The listing builds one solid part. Answer for the finished solid, in the listing's coordinates (mm). Face numbers are marked on the shaded views. Coordinates: 2 decimals unless noted, no trailing zeros. Order: outer loops, then holes, each group sorted by start corner. A loop starts at its lowest first (then second) coordinate and runs counter-clockwise, first axis right, second up. Notation, with made-up numbers: (60.25, -12.75) -> (112.25, -12.75) arc R22 cw to (112.25, 10.25) -> close; hole circle Ø9 at (89, 42). An arc over 180 degrees is marked (long way). Return JSON: item names as keys, results as strings.
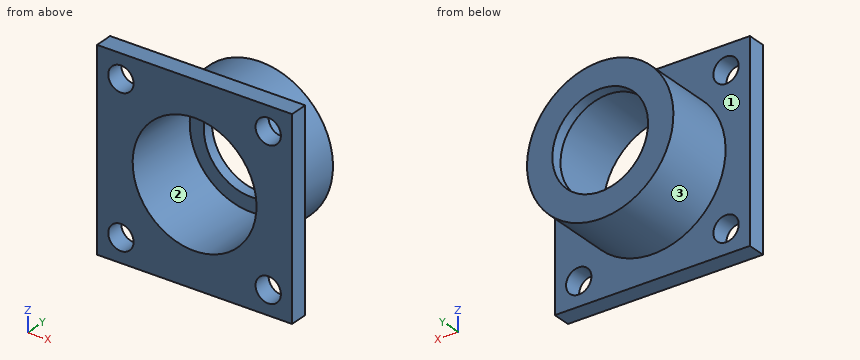
```python
from build123d import *

# Parameters (mm, degrees)
M4_CLEARANCE_HOLE1_D = 4.5
SKETCH5_W            = 85.847558644
SKETCH5_H            = 65.066287946
SKETCH5_W_2          = 34.648232278
SKETCH5_H_2          = 34.648232278
CUT_EXTRUDE2_DEPTH   = 10


with BuildPart() as part:
    # Sketch1 → Revolve1 (revolve)
    with BuildSketch(Plane.XY, mode=Mode.PRIVATE) as revolve1_sk:
        Polygon((-24.5, 0), (-11, 0), (-11, 14), (-8.5, 14), (-8.5, 16), (-13, 16), (-13, 3.2), (-24.5, 3.2), align=None)
    revolve(revolve1_sk.sketch.rotate(Axis((0, 31.465116279, 0), (0, -1, 0)), 270), axis=Axis((0, 31.465116279, 0), (0, -1, 0)))

    # M4 Clearance Hole1 (through all)
    with Locations(Plane(origin=(0, 3.2, 0), x_dir=(1, 0, 0), z_dir=(0, 1, 0))):
        with Locations((-13.081475452, -13.081475452), (-13.081475452, 13.081475452), (13.081475452, 13.081475452), (13.081475452, -13.081475452)):
            Hole(M4_CLEARANCE_HOLE1_D / 2)

    # Sketch5 → Cut-Extrude2 (cut)
    with BuildSketch(Plane(origin=(0, 3.2, 0), x_dir=(1, 0, 0), z_dir=(0, 1, 0))):
        Rectangle(SKETCH5_W, SKETCH5_H)
        Rectangle(SKETCH5_W_2, SKETCH5_H_2, mode=Mode.SUBTRACT)
    extrude(amount=-CUT_EXTRUDE2_DEPTH, mode=Mode.SUBTRACT)


solid = part.part
```
Item 1: The part is cut by section A-A on z = 0. Determine the outline of the cut face in (x, y), plus the area to 3 significant figures.
Answer list:
{"outline": "(-17.32, 0) -> (-11, 0) -> (-11, 14) -> (-8.5, 14) -> (-8.5, 16) -> (-13, 16) -> (-13, 3.2) -> (-17.32, 3.2) -> close; (8.5, 14) -> (11, 14) -> (11, 0) -> (17.32, 0) -> (17.32, 3.2) -> (13, 3.2) -> (13, 16) -> (8.5, 16) -> close", "area": "102 mm2"}
Item 2: The part is cut by section C-C on z = -13.5. Determine the outline of the cut face in (x, y), plus the area to 3 significant figures.
Answer list:
{"outline": "(-17.32, 0) -> (-15.29, 0) -> (-15.29, 3.2) -> (-17.32, 3.2) -> close; (-10.87, 0) -> (10.87, 0) -> (10.87, 3.2) -> (-10.87, 3.2) -> close; (15.29, 0) -> (17.32, 0) -> (17.32, 3.2) -> (15.29, 3.2) -> close", "area": "82.6 mm2"}
Item 3: Find the intervals of material crossed by probe 1 along Z at (x, y) = (-14.5, 1); probe 2 along Y at (x, z) = (14.5, 1.5); probe 3 along Z at (x, y) = (-6.5, 1), in increasing order.
Answer list:
{"probe 1": "-17.32 to -14.83, -11.33 to 11.33, 14.83 to 17.32", "probe 2": "0 to 3.2", "probe 3": "-17.32 to -8.87, 8.87 to 17.32"}
Item 4: The part is cut by section D-D on y = 2.5. Determine the outline of the cut face in (x, z), plus the area to 3 significant figures.
Answer list:
{"outline": "(-17.32, -17.32) -> (17.32, -17.32) -> (17.32, 17.32) -> (-17.32, 17.32) -> close; hole circle Ø4.5 at (-13.08, -13.08); hole circle Ø4.5 at (-13.08, 13.08); hole circle Ø22 at (0, 0); hole circle Ø4.5 at (13.08, -13.08); hole circle Ø4.5 at (13.08, 13.08)", "area": "757 mm2"}
Item 5: Determine the mould class of the marked faces 1, 2 and 3 for opening direction X: pulls with the +X half, pulls with the -X half, needs draft (parallel to the pull), parting line crosses it, or undercut.
Answer list:
{"face 1": "needs draft", "face 2": "undercut", "face 3": "parting line crosses it"}
Item 6: Flat-ended cylindrical pins translate along their axes: pin 1 (3.5 mm diameter, centred on x = -13.08, z = -13.08, fed in from +Y); pin 2 (8 mm diameter, centred on x = -4, y = 3.5, fed in from +Z); pin 3 (6 mm diameter, centred on x = 13.08, z = 13.08, fed in from +Y); pin 4 (5 mm diameter, centred on y = 10, z = 1, fed in from +X). Find the tip coordinate at first contact, or state that the pin passes through.
Answer list:
{"pin 1": "through", "pin 2": "z = 17.32", "pin 3": "y = 3.2", "pin 4": "x = 13"}
Item 7: The part is cut by section B-B on x = 0. Determine the outline of the cut face in (y, z).
Answer list:
{"outline": "(0, -17.32) -> (3.2, -17.32) -> (3.2, -13) -> (16, -13) -> (16, -8.5) -> (14, -8.5) -> (14, -11) -> (0, -11) -> close; (0, 11) -> (14, 11) -> (14, 8.5) -> (16, 8.5) -> (16, 13) -> (3.2, 13) -> (3.2, 17.32) -> (0, 17.32) -> close"}
